Autodesk Inventor part; units mm, degrees
ref_plane "YZ Plane" through (0, 0, 0) normal (1, 0, 0) x (0, 1, 0)
ref_plane "XZ Plane" through (0, 0, 0) normal (0, 1, 0) x (-1, 0, 0)
ref_plane "XY Plane" through (0, 0, 0) normal (0, 0, 1) x (1, 0, 0)
sketch "Sketch2" plane through (0, 0, 0) normal (0, 0, 1) x (1, 0, 0)
  line L0 (-30, 11.5) -> (-30, -11.5)
  line L1 (-30, -11.5) -> (-10, -11.5)
  line L2 (-10, -11.5) -> (-10, 8.5)
  line L3 (-10, 8.5) -> (10, 8.5)
  line L4 (10, 8.5) -> (10, -11.5)
  line L5 (10, -11.5) -> (30, -11.5)
  line L6 (30, -11.5) -> (30, 11.5)
  line L7 (30, 11.5) -> (-30, 11.5)
  point P0 (0, 0)
  point P1 (0, 11.5)
  point P2 (30, 0)
  dimension "d6" = 23
  dimension "d7" = 20
  dimension "d8" = 20
extrude "Extrusion1" add sketch "Sketch2" along normal blind 3
sketch "Sketch3" plane through (0, 0, 3) normal (0, 0, 1) x (1, 0, 0)
  line L0 (30, 11.5) -> (-30, 11.5)
  line L1 (-13, 11.5) -> (-30, -8.5)
  line L2 (-30, 11.5) -> (-30, -11.5)
  line L3 (-30, 11.5) -> (-13, 11.5)
  line L4 (-10, -11.5) -> (-10, 8.5)
  line L5 (13, 11.5) -> (30, -8.5)
  line L6 (30, -11.5) -> (30, 11.5)
  line L7 (10, 8.5) -> (10, -11.5)
  line L8 (10, -11.5) -> (30, -11.5)
  point P0 (0, 0)
  dimension "d11" = 3
  dimension "d12" = 3
  dimension "d13" = 3
  dimension "d14" = 3
extrude "Extrusion2" cut sketch "Sketch3" against normal through all
sketch "Sketch4" plane through (0, 0, 3) normal (0, 0, 1) x (1, 0, 0)
  line L0 (-30, -8.5) -> (-30, -11.5)
  line L1 (-30, -8.5) -> (-13, -8.5)
  line L2 (13, 11.5) -> (-13, 11.5)
  line L3 (-13, -8.5) -> (-13, 11.5)
  line L4 (30, -11.5) -> (30, -8.5)
  line L5 (30, -8.5) -> (13, -8.5)
  line L6 (13, -8.5) -> (13, 11.5)
  line L7 (30, -8.5) -> (13, 11.5)
  line L8 (13, 11.5) -> (-13, 11.5)
  line L9 (-13, 11.5) -> (-30, -8.5)
  line L10 (-30, -8.5) -> (-30, -11.5)
  line L11 (-30, -11.5) -> (-10, -11.5)
  line L12 (-10, -11.5) -> (-10, 8.5)
  line L13 (-10, 8.5) -> (10, 8.5)
  line L14 (10, 8.5) -> (10, -11.5)
  line L15 (10, -11.5) -> (30, -11.5)
  line L16 (30, -11.5) -> (30, -8.5)
  point P0 (0, 0)
  dimension "d17" = 90
  dimension "d20" = 90
extrude "Extrusion3" add sketch "Sketch4" along normal blind 17 contours L1 L3 L2 L6 L5 L4 L15 L14 L13 L12 L11 L0
sketch "Sketch5" plane through (-13, -8.5, 3) normal (-1, 0, 0) x (0, 0, 1)
  line L0 (-3, 17) -> (17, 17)
  line L1 (17, 20) -> (17, 0)
  point P0 (-3, 8.5)
  point P1 (12, 7)
  dimension "d23" = 10
  dimension "d24" = 5
hole "Hole1" at (-13, -1.5, 15) direction (1, 0, 0) diameter 4.5 end through all
sketch "Sketch6" plane through (-30, -8.5, 3) normal (0, 1, 0) x (1, 0, 0)
  line L0 (17, -17) -> (0, -17)
  line L1 (0, 0) -> (0, -17)
  line L2 (60, 0) -> (60, -17)
  point P0 (30, 3)
  point P1 (6, -7)
  point P2 (54, -7)
  dimension "d32" = 10
  dimension "d33" = 6
  dimension "d34" = 6
hole "Hole2" at (-24, -8.5, 10) at (24, -8.5, 10) direction (0, -1, 0) diameter 4.5 end through all
properties part number "Horizontal Support Bracket"
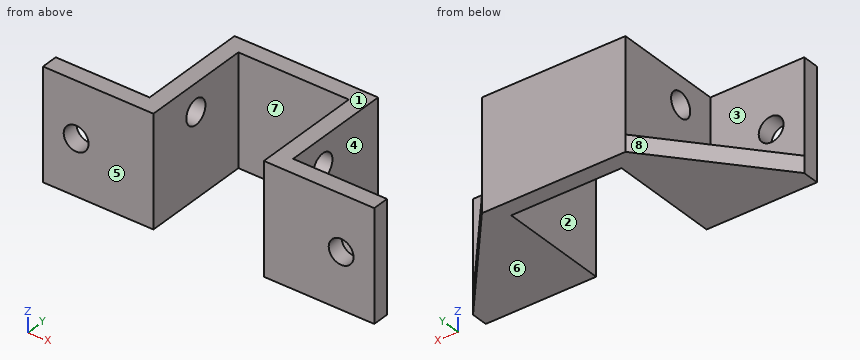
Work out the finished part from the listing and answer in its coordinate system (mm). Face numbers are marked on the shaded views. A direction names the side the tool comes from. Round coordinates to 2 decimals unless told otherwise and drop trailing zeros. Write each loop counter-clockwise with the first axis right and the second up, starting at its lowest first coordinate (ties: lowest second). Pieces come first, ordered by that corner, then holes. Notation, with made-up numbers: (28, 46) - (79, 46) arc R20 cw to (79, 54) - close; hole circle Ø7 at (49.5, 68). An arc over 180 degrees is marked (long way). Answer in a Markdown table with one row per item. Add a question column.
1. Find the intervals of material crossed by line 1 along X through (y, z) = (-4.75, 19); line 2 along Z through (x, y) = (-24, -10.9); line 3 along X through (y, z) = (-10.05, 10), in increasing order. Write a range as from..to.
2. For the marked faces 1, 2, 3, 4 and 5, determine the directions among +Z, -Z, +X, -X, +Y, -Y from which every point of the face is accessible in a straight line to the end or side of a thin tool.
3. Given pin 1 (6 mm diameter, centred on x = -4, z = 15, fed in from -Y); pin 2 (6 mm diameter, centred on y = 1, z = 12.5, fed in from +X); pin 3 (1.5 mm diameter, centred on x = 14.5, z = 5, fed in from +Y); pin 4 (3.5 mm diameter, centred on x = -24, z = 10, fed in from -Y), each flat-ended and moving along its own axis, determine where each tip first touches the part or whether it passes through.
4. A cutting plane is placed at B-B, the plane z = 15. Determine the outline of the cut face in (x, y).
5. A cutting plane is placed at C-C, the plane x = 24. Determine the outline of the cut face in (y, z), and give its area (3 significant figures).
6. A cutting plane is placed at A-A, the plane y = -1.5. Determine the outline of the cut face in (x, z), and give its area (3 significant figures).
7. The mould has two halves that part along X. Classify the marked faces 6, 7 and 8: +X half, -X half, draft (parallel to the pull), parting line (faces both ways), or undercut.
8. A cutting plane is placed at D-D, the plane y = -5. Determine the outline of the cut face in (x, z) (3 decimals), and give its area (3 significant figures).
Worked out:
| question | item | result |
|---|---|---|
| 1 | line 1 | -13..-10, 10..13 |
| 1 | line 2 | 0..7.75, 12.25..20 |
| 1 | line 3 | -30..-26.25, -21.75..-10, 10..21.75, 26.25..30 |
| 2 | face 1 | +Z, +X, -X, +Y, -Y |
| 2 | face 2 | +Z, -Z, -Y |
| 2 | face 3 | +Z, -X, +Y |
| 2 | face 4 | +Z, +X, +Y |
| 2 | face 5 | +Z, -Z, +X, -X, -Y |
| 3 | pin 1 | y = 8.5 |
| 3 | pin 2 | x = 13 |
| 3 | pin 3 | y = -8.5 |
| 3 | pin 4 | through |
| 4 | outline | (-30, -11.5) - (-10, -11.5) - (-10, -3.75) - (-13, -3.75) - (-13, -8.5) - (-30, -8.5) - close; (-13, 0.75) - (-10, 0.75) - (-10, 8.5) - (10, 8.5) - (10, 0.75) - (13, 0.75) - (13, 11.5) - (-13, 11.5) - close; (10, -11.5) - (30, -11.5) - (30, -8.5) - (13, -8.5) - (13, -3.75) - (10, -3.75) - close |
| 5 | outline | (-11.5, 0) - (-1.44, 0) - (-1.44, 3) - (-8.5, 3) - (-8.5, 7.75) - (-11.5, 7.75) - close; (-11.5, 12.25) - (-8.5, 12.25) - (-8.5, 20) - (-11.5, 20) - close |
| 5 | area | 67.7 mm^2 |
| 6 | outline | (-24.05, 0) - (-10, 0) - (-10, 12.75) - (-13, 12.75) - (-13, 3) - (-24.05, 3) - close; (-13, 17.25) - (-10, 17.25) - (-10, 20) - (-13, 20) - close; (10, 0) - (24.05, 0) - (24.05, 3) - (13, 3) - (13, 12.75) - (10, 12.75) - close; (10, 17.25) - (13, 17.25) - (13, 20) - (10, 20) - close |
| 6 | area | 159 mm^2 |
| 7 | face 6 | draft |
| 7 | face 7 | undercut |
| 7 | face 8 | -X half |
| 8 | outline | (-27.025, 0) - (-10, 0) - (-10, 20) - (-13, 20) - (-13, 3) - (-27.025, 3) - close; (10, 0) - (27.025, 0) - (27.025, 3) - (13, 3) - (13, 20) - (10, 20) - close |
| 8 | area | 204 mm^2 |
